Source: CAD feature listing. Evaluate the final solid. Frame: model axes, mm. Face numbers are marked on the shaded views. A direction names the side the tool comes from. Round coordinates to 2 decimals unless told otherwise and drop trailing zeros. Write each loop counter-clockwise with the first axis right and the second up, starting at its lowest first coordinate (ties: lowest second). Pieces come first, ordered by that corner, then holes.
from build123d import *

# Parameters (mm, degrees)
BOSS_EXTRUDE1_DEPTH = 7
FILLET1_R           = 5
FILLET2_R           = 10
CUT_EXTRUDE1_REACH  = 131.101
SKETCH3_R           = 2.5
BOSS_EXTRUDE2_DEPTH = 6
SKETCH7_W           = 4
SKETCH7_H           = 10
BOSS_EXTRUDE3_DEPTH = 27
SKETCH8_R           = 1.5
CUT_EXTRUDE2_DEPTH  = 10
BOSS_EXTRUDE4_DEPTH = 7
BOSS_EXTRUDE5_DEPTH = 7
BOSS_EXTRUDE6_DEPTH = 38.5
SKETCH14_R          = 2
CUT_EXTRUDE3_DEPTH  = 10
CUT_EXTRUDE4_START  = -10
SKETCH15_R          = 2
CUT_EXTRUDE4_DEPTH  = 10


with BuildPart() as part:
    # Sketch1 → Boss-Extrude1 (new body)
    with BuildSketch(Plane(origin=(0, 0, 0), x_dir=(1, 0, 0), z_dir=(0, 1, 0))):
        Polygon((75.055534995, 0), (-54.848275573, 75), (-104.848275573, 75), (-104.848275573, -75), (-54.848275573, -75), align=None)
    extrude(amount=BOSS_EXTRUDE1_DEPTH)

    # Fillet1
    fillet1_edges = [part.edges().sort_by_distance(p)[0] for p in [
        (75.055534995, 3.5, 0),
    ]]
    fillet(fillet1_edges, radius=FILLET1_R)

    # Fillet2
    fillet2_edges = [part.edges().sort_by_distance(p)[0] for p in [
        (-54.848275573, 3.5, 75),
        (-54.848275573, 3.5, -75),
    ]]
    fillet(fillet2_edges, radius=FILLET2_R)

    # Sketch3 → Cut-Extrude1 (cut, up to next)
    with BuildSketch(Plane(origin=(0, 7, 0), x_dir=(1, 0, 0), z_dir=(0, 1, 0)), mode=Mode.PRIVATE) as cut_extrude1_sk1:
        with Locations(Location((-89.848275573, 60, 0), (0, 0, 270))):
            Circle(SKETCH3_R)
    cut_extrude1_tool1 = extrude(cut_extrude1_sk1.sketch, amount=-CUT_EXTRUDE1_REACH, mode=Mode.PRIVATE) & part.part
    # Sketch3 → Cut-Extrude1 (cut, up to next)
    with BuildSketch(Plane(origin=(0, 7, 0), x_dir=(1, 0, 0), z_dir=(0, 1, 0)), mode=Mode.PRIVATE) as cut_extrude1_sk2:
        with Locations(Location((-89.848275573, -60, 0), (0, 0, 270))):
            Circle(SKETCH3_R)
    cut_extrude1_tool2 = extrude(cut_extrude1_sk2.sketch, amount=-CUT_EXTRUDE1_REACH, mode=Mode.PRIVATE) & part.part
    add(cut_extrude1_tool1.solids().sort_by_distance((-89.848276, 7, -60))[0], mode=Mode.SUBTRACT)
    add(cut_extrude1_tool2.solids().sort_by_distance((-89.848276, 7, 60))[0], mode=Mode.SUBTRACT)

    # Sketch6 → Boss-Extrude2 (add)
    with BuildSketch(Plane(origin=(0, 7, 0), x_dir=(1, 0, 0), z_dir=(0, 1, 0))):
        with BuildLine():
            ThreePointArc((-14.848275573, 17.5), (-15.732159049, 19.633883476), (-13.598275573, 18.75))
            Line((-13.598275573, 18.75), (-12.348275573, 18.75))
            ThreePointArc((-12.348275573, 18.75), (-16.616042526, 20.517766953), (-14.848275573, 16.25))
            Line((-14.848275573, 16.25), (-14.848275573, 17.5))
        make_face()
        with BuildLine():
            Line((-12.348275573, 18.75), (-13.598275573, 18.75))
            ThreePointArc((-13.598275573, 18.75), (-13.964392097, 17.866116524), (-14.848275573, 17.5))
            Line((-14.848275573, 17.5), (-14.848275573, 16.25))
            ThreePointArc((-14.848275573, 16.25), (-13.08050862, 16.982233047), (-12.348275573, 18.75))
        make_face()
        with BuildLine():
            ThreePointArc((23.901724427, 18.75), (23.535607903, 17.866116524), (22.651724427, 17.5))
            Line((22.651724427, 17.5), (22.651724427, 16.25))
            ThreePointArc((22.651724427, 16.25), (24.41949138, 16.982233047), (25.151724427, 18.75))
            ThreePointArc((25.151724427, 18.75), (22.651724427, 21.25), (20.151724427, 18.75))
            Line((20.151724427, 18.75), (21.401724427, 18.75))
            ThreePointArc((21.401724427, 18.75), (22.651724427, 20), (23.901724427, 18.75))
        make_face()
        with BuildLine():
            Line((22.651724427, 16.25), (22.651724427, 17.5))
            ThreePointArc((22.651724427, 17.5), (21.767840951, 17.866116524), (21.401724427, 18.75))
            Line((21.401724427, 18.75), (20.151724427, 18.75))
            ThreePointArc((20.151724427, 18.75), (20.883957474, 16.982233047), (22.651724427, 16.25))
        make_face()
        with BuildLine():
            ThreePointArc((22.651724427, -16.25), (20.883957474, -16.982233047), (20.151724427, -18.75))
            Line((20.151724427, -18.75), (21.401724427, -18.75))
            ThreePointArc((21.401724427, -18.75), (21.767840951, -17.866116524), (22.651724427, -17.5))
            Line((22.651724427, -17.5), (22.651724427, -16.25))
        make_face()
        with BuildLine():
            Line((21.401724427, -18.75), (20.151724427, -18.75))
            ThreePointArc((20.151724427, -18.75), (22.651724427, -21.25), (25.151724427, -18.75))
            ThreePointArc((25.151724427, -18.75), (24.41949138, -16.982233047), (22.651724427, -16.25))
            Line((22.651724427, -16.25), (22.651724427, -17.5))
            ThreePointArc((22.651724427, -17.5), (23.535607903, -17.866116524), (23.901724427, -18.75))
            ThreePointArc((23.901724427, -18.75), (22.651724427, -20), (21.401724427, -18.75))
        make_face()
        with BuildLine():
            ThreePointArc((-14.848275573, -17.5), (-13.964392097, -17.866116524), (-13.598275573, -18.75))
            Line((-13.598275573, -18.75), (-12.348275573, -18.75))
            ThreePointArc((-12.348275573, -18.75), (-13.08050862, -16.982233047), (-14.848275573, -16.25))
            Line((-14.848275573, -16.25), (-14.848275573, -17.5))
        make_face()
        with BuildLine():
            Line((-12.348275573, -18.75), (-13.598275573, -18.75))
            ThreePointArc((-13.598275573, -18.75), (-15.732159049, -19.633883476), (-14.848275573, -17.5))
            Line((-14.848275573, -17.5), (-14.848275573, -16.25))
            ThreePointArc((-14.848275573, -16.25), (-16.616042526, -20.517766953), (-12.348275573, -18.75))
        make_face()
    extrude(amount=BOSS_EXTRUDE2_DEPTH)

    # Sketch7 → Boss-Extrude3 (add)
    with BuildSketch(Plane(origin=(0, 7, 0), x_dir=(1, 0, 0), z_dir=(0, 1, 0))):
        Polygon((-89.848275573, 5), (-85.848275573, 5), (-85.848275573, 17), (-93.848275573, 17), (-93.848275573, -17), (-85.848275573, -17), (-85.848275573, -5), (-89.848275573, -5), align=None)
        with Locations((-87.848275573, 0)):
            Rectangle(SKETCH7_W, SKETCH7_H)
    extrude(amount=BOSS_EXTRUDE3_DEPTH)

    # Sketch8 → Cut-Extrude2 (cut)
    with BuildSketch(Plane(origin=(0, 34, 0), x_dir=(1, 0, 0), z_dir=(0, 1, 0))):
        with Locations(Location((-89.848275573, -5, 0), (0, 0, 270))):
            Circle(SKETCH8_R)
        with Locations(Location((-89.848275573, 5, 0), (0, 0, 270))):
            Circle(SKETCH8_R)
    extrude(amount=-CUT_EXTRUDE2_DEPTH, mode=Mode.SUBTRACT)

    # Sketch7<4> → Boss-Extrude4 (add)
    with BuildSketch(Plane(origin=(0, 7, 0), x_dir=(1, 0, 0), z_dir=(0, 1, 0))):
        Polygon((-45.848275573, -17), (-37.848275573, -17), (-37.848275573, -7), (-45.348275573, -7), (-45.348275573, -10.506475343), (-55.348275573, -10.506475343), (-55.348275573, -17), align=None)
    extrude(amount=BOSS_EXTRUDE4_DEPTH)

    # Sketch7<5> → Boss-Extrude5 (add)
    with BuildSketch(Plane(origin=(0, 7, 0), x_dir=(1, 0, 0), z_dir=(0, 1, 0))):
        Polygon((-45.848275573, 17), (-37.848275573, 17), (-37.848275573, 7), (-45.348275573, 7), (-45.348275573, 10.493524657), (-55.348275573, 10.493524657), (-55.348275573, 17), align=None)
    extrude(amount=BOSS_EXTRUDE5_DEPTH)

    # Sketch11 → Boss-Extrude6 (add)
    with BuildSketch(Plane(origin=(0, 7, 0), x_dir=(1, 0, 0), z_dir=(0, 1, 0))):
        with BuildLine():
            Line((-104.848275573, 75), (-104.848275573, -75))
            Line((-104.848275573, -75), (-57.527767497, -75))
            ThreePointArc((-57.527767497, -75), (-54.939577046, -74.659258263), (-52.527767497, -73.660254038))
            Line((-52.527767497, -73.660254038), (67.555534995, -4.330127019))
            ThreePointArc((67.555534995, -4.330127019), (70.055534995, 0), (67.555534995, 4.330127019))
            Line((67.555534995, 4.330127019), (-52.527767497, 73.660254038))
            ThreePointArc((-52.527767497, 73.660254038), (-54.939577046, 74.659258263), (-57.527767497, 75))
            Line((-57.527767497, 75), (-104.848275573, 75))
        make_face()
        with BuildLine():
            ThreePointArc((-55.027767497, 69.330127019), (-56.233672272, 69.829629131), (-57.527767497, 70))
            Line((-57.527767497, 70), (-99.848275573, 70))
            Line((-99.848275573, 70), (-99.848275573, -70))
            Line((-99.848275573, -70), (-57.527767497, -70))
            ThreePointArc((-57.527767497, -70), (-56.233672272, -69.829629131), (-55.027767497, -69.330127019))
            Line((-55.027767497, -69.330127019), (65.055534995, 0))
            Line((65.055534995, 0), (-55.027767497, 69.330127019))
        make_face(mode=Mode.SUBTRACT)
    extrude(amount=BOSS_EXTRUDE6_DEPTH)

    # Sketch14 → Cut-Extrude3 (cut)
    with BuildSketch(Plane.XY.offset(75)):
        with Locations((-95.848275573, 10)):
            Circle(SKETCH14_R)
    extrude(amount=-CUT_EXTRUDE3_DEPTH, mode=Mode.SUBTRACT)

    # Sketch15 → Cut-Extrude4 (cut)
    with BuildSketch(Plane(origin=(0, 0, -75), x_dir=(-1, 0, 0), z_dir=(0, 0, -1)).offset(CUT_EXTRUDE4_START)):
        with Locations(Location((95.848275573, 10, 0), (0, 0, 180))):
            Circle(SKETCH15_R)
    extrude(amount=CUT_EXTRUDE4_DEPTH, mode=Mode.SUBTRACT)


solid = part.part
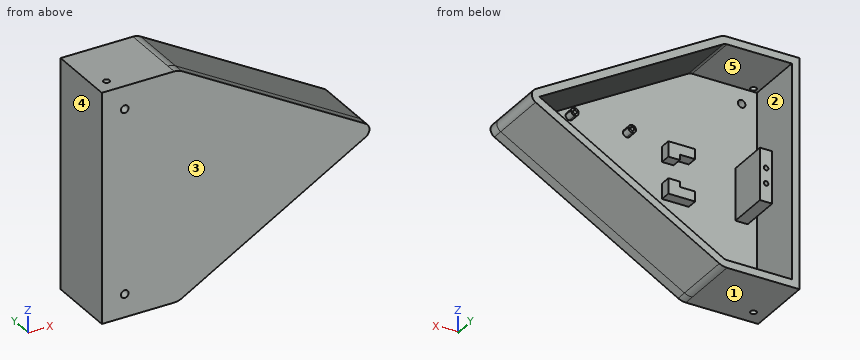
1) Material intervals for line 1 (Z direction, x = -62, y = 28.5); line 2 (X direction, y = 9.1, z = 18.75); line 3 (X direction, y = 29, z = 5), sorted ascending.
Taken from the geometry:
line 1: z = -75 to -70, 70 to 75
line 2: x = -104.85 to -99.85, -17.35 to -16.1, -13.6 to -12.35, 20.15 to 21.4, 23.9 to 25.15, 32.58 to 42.58
line 3: x = -104.85 to -99.85, -93.85 to -91.35, -88.35 to -85.85, 56.4 to 66.4
2) Section query C-C on z = -60. Return the cut outline in (x, y), then the cut area to 3 significant figures.
Taken from the geometry:
outline: (-104.85, 0) - (-92.35, 0) - (-92.35, 7) - (-99.85, 7) - (-99.85, 45.5) - (-104.85, 45.5) - close; (-87.35, 0) - (-28.87, 0) - (-28.87, 45.5) - (-38.87, 45.5) - (-38.87, 7) - (-87.35, 7) - close
area: 1,070 mm2
3) Section query D-D on y = 37. Return the cut outline in (x, z).
Taken from the geometry:
outline: (-104.85, -75) - (-57.53, -75) arc R10 ccw to (-52.53, -73.66) - (67.56, -4.33) arc R5 ccw to (67.56, 4.33) - (-52.53, 73.66) arc R10 ccw to (-57.53, 75) - (-104.85, 75) - close; hole (-99.85, -70) - (-57.53, -70) arc R5 ccw to (-55.03, -69.33) - (65.06, 0) - (-55.03, 69.33) arc R5 ccw to (-57.53, 70) - (-99.85, 70) - close
4) Section query A-A on y = 10. State how many separate pieces and enclosed holes the cut face has, then the cut area to 3 significant figures.
Taken from the geometry:
separate pieces: 9
enclosed holes: 4
area: 3,200 mm2
5) Contact query for flat-ended pins moving along their axis: P1, Ø3.5, axis at x = -47, y = 10, coming from the -Z side; P2, Ø5.5, axis at x = -53, y = 9, coming from the -Z side; P3, Ø0.8, axis at x = 22.5, z = -19, coming from the +Y side. Output: stop coordinate, or through.
Taken from the geometry:
P1: stops at z = -71.48
P2: stops at z = -74.84
P3: stops at y = 7
6) Pull-direction query (Z, two-part tool) for the marked faces 1, 2 and 3; classes: released by +Z, released by -Z, zero draft, split by the parting line, or undercut.
Taken from the geometry:
face 1: released by -Z
face 2: undercut
face 3: zero draft
7) Section query B-B on x = -62. Return the cut outline in (y, z).
Taken from the geometry:
outline: (0, -75) - (45.5, -75) - (45.5, -70) - (7, -70) - (7, 70) - (45.5, 70) - (45.5, 75) - (0, 75) - close
8) Reachability of the marked faces 4 and 5 from +Z, -Z, +X, -X, +Y, -Y: full face, straight path, thin tool, end or side. Return the list, or none.
Taken from the geometry:
face 4: +Z, -Z, -X, +Y, -Y
face 5: +Y
